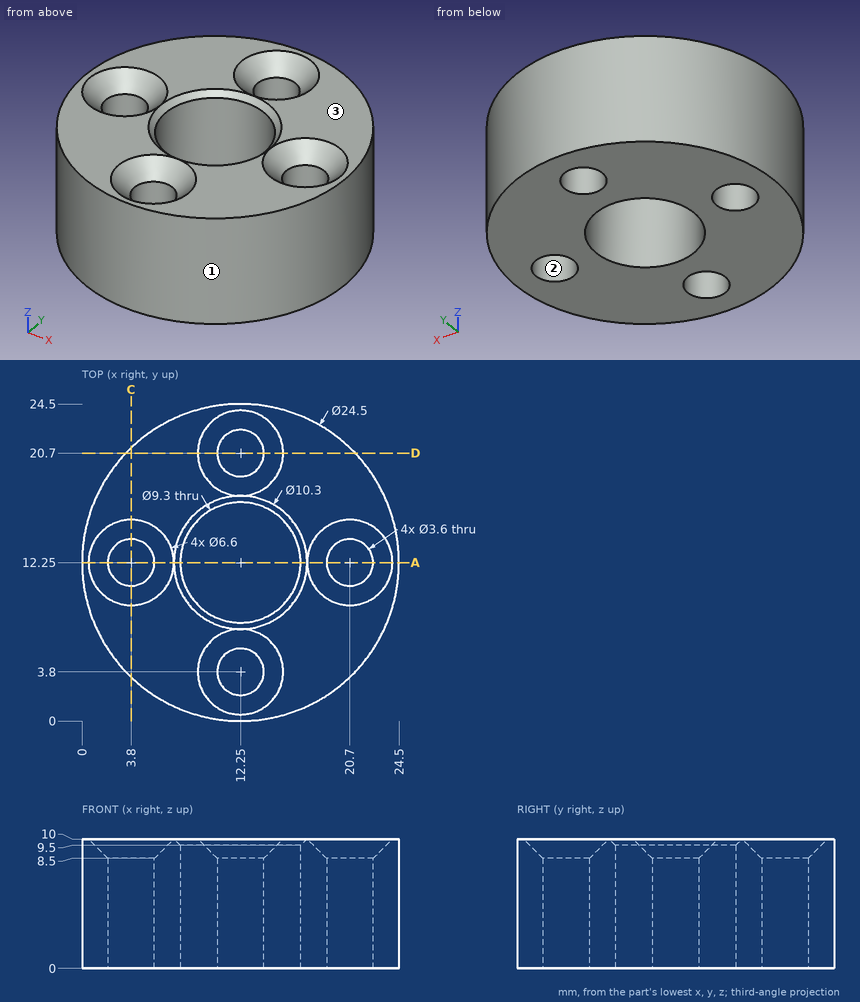
Can you work these out from the drawing? Everything is in mm from the part's minimum corner. Give positions to 0.01 mm unless a question says otherwise; leave off trailing zeros. Order: outer loops, then holes, each group sorted by start corner. A loop starts at its lowest first (then second) coordinate and runs counter-clockwise, first axis right, second up. Notation, with made-up numbers: (56, 25) -> (62, 25) arc R7 ccw to (62, 35) -> close; hole circle Ø6 at (54, 76). An arc over 180 degrees is marked (long way). Return JSON: item names as keys, results as strings.
1. I need wall thicknesses on line 1 (Y direction, x = 12.25, z = 7); line 2 (X direction, y = 19.25, z = 1.5); line 3 (Y direction, x = 3.5, z = 3.25). Which ranges of each line are inside material? Lowest first, please. Write a range as from..to.
Answer list:
{"line 1": "y = 0..2, 5.6..7.6, 16.9..18.9, 22.5..24.5", "line 2": "x = 2.2..11.18, 13.32..22.3", "line 3": "y = 3.68..10.48, 14.02..20.82"}
2. Imagine slicing it at C-C on x = 3.8. List the corners of the cut face in (y, z) for me, then the cut area to 3 significant figures.
Answer list:
{"outline": "(3.38, 0) -> (10.45, 0) -> (10.45, 8.5) -> (8.95, 10) -> (3.38, 10) -> close; (14.05, 0) -> (21.12, 0) -> (21.12, 10) -> (15.55, 10) -> (14.05, 8.5) -> close", "area": "139 mm2"}
3. For pin 1 Ø3 at (y, z) = (18, 5.5) entering from -X; pin 2 Ø6 at (y, z) = (8, 8.5) entering from +X; pin 3 Ø6 at (y, z) = (2.5, 7) entering from +X, each with a flat end and sliding along its axis, tell me the tip position at first contact or that it passes through.
Answer list:
{"pin 1": "stops at x = 0.76", "pin 2": "stops at x = 24.44", "pin 3": "stops at x = 22.47"}
4. Imagine slicing it at A-A on y = 12.25. Give the number of separate pieces and of enclosed holes in the cut face, then the cut area to 4 significant figures.
Answer list:
{"separate pieces": "4", "enclosed holes": "0", "area": "75.25 mm2"}
5. Thinking about a two-plate mould opening in Y: for the marked faces 1, 2 and 3, which applies, pulls with the +Y half, pulls with the -Y half, needs draft (parallel to the pull), parting line crosses it, or undercut?
Answer list:
{"face 1": "parting line crosses it", "face 2": "undercut", "face 3": "needs draft"}
